Geometry check sheet. Reference: the model listing, model coordinates, mm. A direction names the side the tool comes from. Give positions to 0.01 mm unless a question says otherwise; leave off trailing zeros. Order: outer loops, then holes, each group sorted by start corner. A loop starts at its lowest first (then second) coordinate and runs counter-clockwise, first axis right, second up. Notation, with made-up numbers: M 75.5,11.25 L 117.5,11.25 A28 cw 117.5,50.25 Z; hole C 86.5,22.5 d6. An arc over 180 degrees is marked long. One line per question, with ' | ' between items. Start each with the question number.
from build123d import *

# Parameters (mm, degrees)
EXTRUDE_2_DEPTH     = 15
SKETCH_2_R          = 2.62067407
CUT_EXTRUDE_1_DEPTH = 74.942500428
FILLET_1_R          = 7
CUT_EXTRUDE_2_REACH = 79.534
SKETCH_3_R          = 3
SKETCH_3_R_2        = 1.5
FILLET_2_R          = 5


with BuildPart() as part:
    # 草图1 → 拉伸-薄壁2 (new, symmetric)
    with BuildSketch(Plane.XY):
        Polygon((-29.774038515, 0), (29.774038515, 0), (29.774038515, 70), (0, 70), (-29.774038515, 70), align=None)
        Polygon((-25.774038515, 4), (25.774038515, 4), (25.774038515, 66), (0, 66), (-25.774038515, 66), align=None, mode=Mode.SUBTRACT)
    extrude(amount=EXTRUDE_2_DEPTH, both=True)

    # 草图2 → 切除-拉伸1 (cut, through all)
    with BuildSketch(Plane(origin=(0, 66, 0), x_dir=(-1, 0, 0), z_dir=(0, -1, 0))):
        with Locations(Location((-15, 0, 0), (0, 0, 90))):
            Circle(SKETCH_2_R)
        with Locations(Location((15, 0, 0), (0, 0, 90))):
            Circle(SKETCH_2_R)
    extrude(amount=-CUT_EXTRUDE_1_DEPTH, mode=Mode.SUBTRACT)

    # 圆角1
    fillet_1_edges = [part.edges().sort_by_distance(p)[0] for p in [
        (-25.774038515, 4, 0),
        (25.774038515, 4, 0),
        (25.774038515, 66, 0),
        (-25.774038515, 66, 0),
    ]]
    fillet(fillet_1_edges, radius=FILLET_1_R)

    # 草图3 → 切除-拉伸2 (cut, up to next)
    with BuildSketch(Plane(origin=(0, 0, 0), x_dir=(1, 0, 0), z_dir=(0, 1, 0)), mode=Mode.PRIVATE) as cut_extrude_2_sk1:
        with Locations(Location((0, 0, 0), (0, 0, 180))):
            Circle(SKETCH_3_R)
    cut_extrude_2_tool1 = extrude(cut_extrude_2_sk1.sketch, amount=CUT_EXTRUDE_2_REACH, mode=Mode.PRIVATE) & part.part
    # 草图3 → 切除-拉伸2 (cut, up to next)
    with BuildSketch(Plane(origin=(0, 0, 0), x_dir=(1, 0, 0), z_dir=(0, 1, 0)), mode=Mode.PRIVATE) as cut_extrude_2_sk2:
        with Locations(Location((-15, 5, 0), (0, 0, 180))):
            Circle(SKETCH_3_R_2)
    cut_extrude_2_tool2 = extrude(cut_extrude_2_sk2.sketch, amount=CUT_EXTRUDE_2_REACH, mode=Mode.PRIVATE) & part.part
    # 草图3 → 切除-拉伸2 (cut, up to next)
    with BuildSketch(Plane(origin=(0, 0, 0), x_dir=(1, 0, 0), z_dir=(0, 1, 0)), mode=Mode.PRIVATE) as cut_extrude_2_sk3:
        with Locations(Location((-5, 5, 0), (0, 0, 180))):
            Circle(SKETCH_3_R_2)
    cut_extrude_2_tool3 = extrude(cut_extrude_2_sk3.sketch, amount=CUT_EXTRUDE_2_REACH, mode=Mode.PRIVATE) & part.part
    # 草图3 → 切除-拉伸2 (cut, up to next)
    with BuildSketch(Plane(origin=(0, 0, 0), x_dir=(1, 0, 0), z_dir=(0, 1, 0)), mode=Mode.PRIVATE) as cut_extrude_2_sk4:
        with Locations(Location((5, 5, 0), (0, 0, 180))):
            Circle(SKETCH_3_R_2)
    cut_extrude_2_tool4 = extrude(cut_extrude_2_sk4.sketch, amount=CUT_EXTRUDE_2_REACH, mode=Mode.PRIVATE) & part.part
    # 草图3 → 切除-拉伸2 (cut, up to next)
    with BuildSketch(Plane(origin=(0, 0, 0), x_dir=(1, 0, 0), z_dir=(0, 1, 0)), mode=Mode.PRIVATE) as cut_extrude_2_sk5:
        with Locations(Location((15, 5, 0), (0, 0, 180))):
            Circle(SKETCH_3_R_2)
    cut_extrude_2_tool5 = extrude(cut_extrude_2_sk5.sketch, amount=CUT_EXTRUDE_2_REACH, mode=Mode.PRIVATE) & part.part
    # 草图3 → 切除-拉伸2 (cut, up to next)
    with BuildSketch(Plane(origin=(0, 0, 0), x_dir=(1, 0, 0), z_dir=(0, 1, 0)), mode=Mode.PRIVATE) as cut_extrude_2_sk6:
        with Locations(Location((-5, -5, 0), (0, 0, 180))):
            Circle(SKETCH_3_R_2)
    cut_extrude_2_tool6 = extrude(cut_extrude_2_sk6.sketch, amount=CUT_EXTRUDE_2_REACH, mode=Mode.PRIVATE) & part.part
    # 草图3 → 切除-拉伸2 (cut, up to next)
    with BuildSketch(Plane(origin=(0, 0, 0), x_dir=(1, 0, 0), z_dir=(0, 1, 0)), mode=Mode.PRIVATE) as cut_extrude_2_sk7:
        with Locations(Location((5, -5, 0), (0, 0, 180))):
            Circle(SKETCH_3_R_2)
    cut_extrude_2_tool7 = extrude(cut_extrude_2_sk7.sketch, amount=CUT_EXTRUDE_2_REACH, mode=Mode.PRIVATE) & part.part
    # 草图3 → 切除-拉伸2 (cut, up to next)
    with BuildSketch(Plane(origin=(0, 0, 0), x_dir=(1, 0, 0), z_dir=(0, 1, 0)), mode=Mode.PRIVATE) as cut_extrude_2_sk8:
        with Locations(Location((15, -5, 0), (0, 0, 180))):
            Circle(SKETCH_3_R_2)
    cut_extrude_2_tool8 = extrude(cut_extrude_2_sk8.sketch, amount=CUT_EXTRUDE_2_REACH, mode=Mode.PRIVATE) & part.part
    # 草图3 → 切除-拉伸2 (cut, up to next)
    with BuildSketch(Plane(origin=(0, 0, 0), x_dir=(1, 0, 0), z_dir=(0, 1, 0)), mode=Mode.PRIVATE) as cut_extrude_2_sk9:
        with Locations(Location((-15, -5, 0), (0, 0, 180))):
            Circle(SKETCH_3_R_2)
    cut_extrude_2_tool9 = extrude(cut_extrude_2_sk9.sketch, amount=CUT_EXTRUDE_2_REACH, mode=Mode.PRIVATE) & part.part
    add(cut_extrude_2_tool1.solids().sort_by_distance((0, 0, 0))[0], mode=Mode.SUBTRACT)
    add(cut_extrude_2_tool2.solids().sort_by_distance((-15, 0, -5))[0], mode=Mode.SUBTRACT)
    add(cut_extrude_2_tool3.solids().sort_by_distance((-5, 0, -5))[0], mode=Mode.SUBTRACT)
    add(cut_extrude_2_tool4.solids().sort_by_distance((5, 0, -5))[0], mode=Mode.SUBTRACT)
    add(cut_extrude_2_tool5.solids().sort_by_distance((15, 0, -5))[0], mode=Mode.SUBTRACT)
    add(cut_extrude_2_tool6.solids().sort_by_distance((-5, 0, 5))[0], mode=Mode.SUBTRACT)
    add(cut_extrude_2_tool7.solids().sort_by_distance((5, 0, 5))[0], mode=Mode.SUBTRACT)
    add(cut_extrude_2_tool8.solids().sort_by_distance((15, 0, 5))[0], mode=Mode.SUBTRACT)
    add(cut_extrude_2_tool9.solids().sort_by_distance((-15, 0, 5))[0], mode=Mode.SUBTRACT)

    # 圆角2
    fillet_2_edges = [part.edges().sort_by_distance(p)[0] for p in [
        (-29.774038515, 0, 0),
        (-29.774038515, 70, 0),
        (29.774038515, 70, 0),
        (29.774038515, 0, 0),
    ]]
    fillet(fillet_2_edges, radius=FILLET_2_R)


solid = part.part
Item 1: Cross-section at D-D, the plane y = 39.5. Record the cut outline in (x, z).
Item 2: Cross-section at C-C, the plane x = 15. Record the cut outline in (y, z), plus the area to 3 significant figures.
Item 3: Material ranges on line 1 along Z through (x, y) = (5, 2.7); line 2 along Y through (x, z) = (-3.5, 10.25); line 3 along X through (y, z) = (17.5, 13.5), recorded low to high.
Item 4: Cross-section at B-B, the plane x = -10.5. Record the cut outline in (y, z), plus the area to 3 significant figures.
Item 5: Cross-section at A-A, the plane z = 5. State how many separate pieces and enclosed holes the cut face has, plus the area to 3 significant figures.
Item 6: Set-up check for faces 4 (the cylindrical face through (16.5, 1.97, -4.93)), 5 (the cylindrical face through (-17.558, 67.972, 0.568)), 6 (the flat face through (25.774, 35, 0)): record each of +Z, -Z, +X, -X, +Y, -Y from which the full face is reachable in a straight line by a thin tool's end or side.
Item 7: Depth check by flat-ended pin: pin 1 (12 mm diameter, centred on x = 17, y = 11.5, fed in from +Z); pin 2 (1.8 mm diameter, centred on x = 15, z = 5, fed in from -Y). Enter the tip coordinate at first touch or a pass-through.
Item 8: Mould release check, pull along X, two halves, no side actions. Record for faces 1 (the cylindrical face through (28.27, 1.426, 0.21)), 2 (the flat face through (-25.774, 35, 0)), 3 (the flat face through (-27, 40, -15)): released by +X, released by -X, zero draft, split by the parting line, or undercut.
Outcome:
1) outline: M -29.77,-15 L -25.77,-15 L -25.77,15 L -29.77,15 Z; M 25.77,-15 L 29.77,-15 L 29.77,15 L 25.77,15 Z
2) outline: M 0,-15 L 4,-15 L 4,-6.5 L 0,-6.5 Z; M 0,-3.5 L 4,-3.5 L 4,3.5 L 0,3.5 Z; M 0,6.5 L 4,6.5 L 4,15 L 0,15 Z; M 66,-15 L 70,-15 L 70,-2.62 L 66,-2.62 Z; M 66,2.62 L 70,2.62 L 70,15 L 66,15 Z | area: 195 mm²
3) line 1: z = -15 to -6.5, -3.5 to 3.5, 6.5 to 15 | line 2: y = 0 to 4, 66 to 70 | line 3: x = -29.77 to -25.77, 25.77 to 29.77
4) outline: M 0,-15 L 4,-15 L 4,15 L 0,15 Z; M 66,-15 L 70,-15 L 70,15 L 66,15 Z | area: 240 mm²
5) separate pieces: 4 | enclosed holes: 0 | area: 945 mm²
6) face 4: -Y | face 5: +Y | face 6: +Z, -Z
7) pin 1: passes through | pin 2: stops at y = 66
8) face 1: released by +X | face 2: undercut | face 3: zero draft
